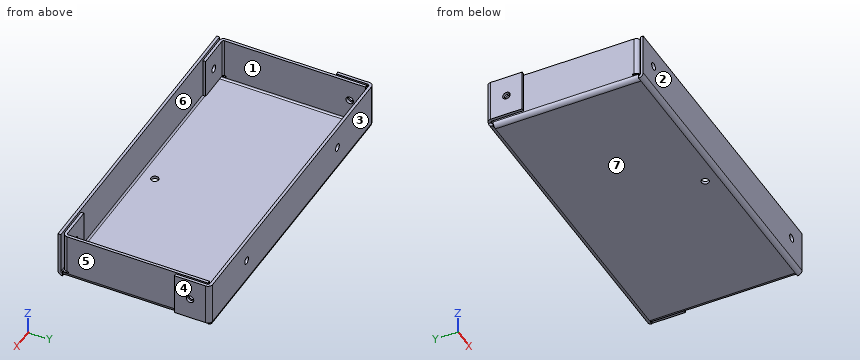
```python
from build123d import *

# Parameters (mm, degrees)
SKETCH1_W                        = 140
SKETCH1_H                        = 70
BASE_FLANGE1_DEPTH               = 1.29
EDGE_FLANGE1_STRIP_W             = 6.684
EDGE_FLANGE1_STRIP_H             = 1.29
EDGE_FLANGE1_STRIP_CUT_DEPTH     = 140
EDGE_FLANGE1_DEPTH               = 140
EDGE_FLANGE2_STRIP_W             = 6.684
EDGE_FLANGE2_STRIP_H             = 1.29
EDGE_FLANGE2_STRIP_CUT_DEPTH     = 140
EDGE_FLANGE2_DEPTH               = 140
EDGE_FLANGE3_STRIP_W             = 6.684
EDGE_FLANGE3_STRIP_H             = 1.29
EDGE_FLANGE3_STRIP_CUT_DEPTH     = 65.896
EDGE_FLANGE3_DEPTH               = 65.896
EDGE_FLANGE4_STRIP_W             = 6.684
EDGE_FLANGE4_STRIP_H             = 1.29
EDGE_FLANGE4_STRIP_CUT_DEPTH     = 65.896
EDGE_FLANGE4_DEPTH               = 65.896
EDGE_FLANGE6_START               = 1.117
EDGE_FLANGE6_DEPTH               = 18.883
EDGE_FLANGE6_2_DEPTH             = 0.645
EDGE_FLANGE6_START_2             = 1.762
EDGE_FLANGE6_3_DEPTH             = 18.238
EDGE_FLANGE8_START               = 1.117
EDGE_FLANGE8_DEPTH               = 18.883
EDGE_FLANGE8_2_DEPTH             = 0.645
EDGE_FLANGE8_START_2             = 1.762
EDGE_FLANGE8_3_DEPTH             = 18.238
M3_CLEARANCE_HOLE1_D             = 3.4
EDGE_FLANGE9_DEPTH               = 19.238
EDGE_FLANGE10_DEPTH              = 19.238
TAP_DRILL_FOR_M4X0_7_TAP1_REACH  = 161.621
TAP_DRILL_FOR_M4X0_7_TAP1_BORE_R = 1.65
M3_CLEARANCE_HOLE3_D             = 3.4
M3_CLEARANCE_HOLE3_DEPTH         = 3.342
M3_CLEARANCE_HOLE4_D             = 3.4


# Read off the part's stored shape, not the designer's step: Edge-Flange6, Edge-Flange8
# Sheet-metal steps are written as plain solids
with BuildPart() as part:
    # Sketch1 → Base-Flange1 (new body)
    with BuildSketch(Plane.XY):
        with Locations((70, 35)):
            Rectangle(SKETCH1_W, SKETCH1_H)
    extrude(amount=-BASE_FLANGE1_DEPTH)

    # Edge-Flange1 strip (across the edge) → Edge-Flange1 strip cut (cut)
    with BuildSketch(Plane(origin=(140, 70, 0), x_dir=(0, -1, 0), z_dir=(-1, 0, 0))):
        with Locations((-1.29, -0.645)):
            Rectangle(EDGE_FLANGE1_STRIP_W, EDGE_FLANGE1_STRIP_H)
    extrude(amount=EDGE_FLANGE1_STRIP_CUT_DEPTH, mode=Mode.SUBTRACT)

    # Edge-Flange1 section (across the edge) → Edge-Flange1 (add)
    with BuildSketch(Plane(origin=(140, 70, 0), x_dir=(0, -1, 0), z_dir=(-1, 0, 0))):
        with BuildLine():
            Line((0, 0.762), (0, 20))
            Line((0, 20), (1.29, 20))
            Line((1.29, 20), (1.29, 0.762))
            ThreePointArc((1.29, 0.762), (1.513184633, 0.223184633), (2.052, 0))
            Line((2.052, 0), (2.052, -1.29))
            ThreePointArc((2.052, -1.29), (0.601016885, -0.688983115), (0, 0.762))
        make_face()
    extrude(amount=EDGE_FLANGE1_DEPTH)

    # Edge-Flange2 strip (across the edge) → Edge-Flange2 strip cut (cut)
    with BuildSketch(Plane.YZ):
        with Locations((-1.29, -0.645)):
            Rectangle(EDGE_FLANGE2_STRIP_W, EDGE_FLANGE2_STRIP_H)
    extrude(amount=EDGE_FLANGE2_STRIP_CUT_DEPTH, mode=Mode.SUBTRACT)

    # Edge-Flange2 section (across the edge) → Edge-Flange2 (add)
    with BuildSketch(Plane.YZ):
        with BuildLine():
            Line((0, 0.762), (0, 20))
            Line((0, 20), (1.29, 20))
            Line((1.29, 20), (1.29, 0.762))
            ThreePointArc((1.29, 0.762), (1.513184633, 0.223184633), (2.052, 0))
            Line((2.052, 0), (2.052, -1.29))
            ThreePointArc((2.052, -1.29), (0.601016885, -0.688983115), (0, 0.762))
        make_face()
    extrude(amount=EDGE_FLANGE2_DEPTH)

    # Edge-Flange3 strip (across the edge) → Edge-Flange3 strip cut (cut)
    with BuildSketch(Plane.XZ.offset(-67.948)):
        with Locations((-1.29, -0.645)):
            Rectangle(EDGE_FLANGE3_STRIP_W, EDGE_FLANGE3_STRIP_H)
    extrude(amount=EDGE_FLANGE3_STRIP_CUT_DEPTH, mode=Mode.SUBTRACT)

    # Edge-Flange3 section (across the edge) → Edge-Flange3 (add)
    with BuildSketch(Plane.XZ.offset(-67.948)):
        with BuildLine():
            Line((0, 0.762), (0, 20))
            Line((0, 20), (1.29, 20))
            Line((1.29, 20), (1.29, 0.762))
            ThreePointArc((1.29, 0.762), (1.513184633, 0.223184633), (2.052, 0))
            Line((2.052, 0), (2.052, -1.29))
            ThreePointArc((2.052, -1.29), (0.601016885, -0.688983115), (0, 0.762))
        make_face()
    extrude(amount=EDGE_FLANGE3_DEPTH)

    # Edge-Flange4 strip (across the edge) → Edge-Flange4 strip cut (cut)
    with BuildSketch(Plane(origin=(140, 2.052, 0), x_dir=(-1, 0, 0), z_dir=(0, 1, 0))):
        with Locations((-1.29, -0.645)):
            Rectangle(EDGE_FLANGE4_STRIP_W, EDGE_FLANGE4_STRIP_H)
    extrude(amount=EDGE_FLANGE4_STRIP_CUT_DEPTH, mode=Mode.SUBTRACT)

    # Edge-Flange4 section (across the edge) → Edge-Flange4 (add)
    with BuildSketch(Plane(origin=(140, 2.052, 0), x_dir=(-1, 0, 0), z_dir=(0, 1, 0))):
        with BuildLine():
            Line((0, 0.762), (0, 20))
            Line((0, 20), (1.29, 20))
            Line((1.29, 20), (1.29, 0.762))
            ThreePointArc((1.29, 0.762), (1.513184633, 0.223184633), (2.052, 0))
            Line((2.052, 0), (2.052, -1.29))
            ThreePointArc((2.052, -1.29), (0.601016885, -0.688983115), (0, 0.762))
        make_face()
    extrude(amount=EDGE_FLANGE4_DEPTH)

    # Edge-Flange6 outline → Edge-Flange6 (cut)
    with BuildSketch(Plane.XY.offset(EDGE_FLANGE6_START)):
        with BuildLine():
            Line((1.29, 2.052), (1.29, 2.198728366))
            ThreePointArc((1.29, 2.198728366), (0.352834322, 2.953547915), (0, 4.104))
            Line((0, 4.104), (0, 2.052))
            Line((0, 2.052), (1.29, 2.052))
        make_face()
    extrude(amount=EDGE_FLANGE6_DEPTH, mode=Mode.SUBTRACT)

    # Edge-Flange6 2 outline → Edge-Flange6 2 (cut)
    with BuildSketch(Plane.XY.offset(EDGE_FLANGE6_START)):
        with BuildLine():
            ThreePointArc((0, 4.104), (0.352834322, 2.953547915), (1.29, 2.198728366))
            Line((1.29, 2.198728366), (1.29, 4.749))
            Line((1.29, 4.749), (0, 4.749))
            Line((0, 4.749), (0, 4.104))
        make_face()
    extrude(amount=EDGE_FLANGE6_2_DEPTH, mode=Mode.SUBTRACT)

    # Edge-Flange6 3 outline → Edge-Flange6 3 (add)
    with BuildSketch(Plane.XY.offset(EDGE_FLANGE6_START_2)):
        with BuildLine():
            Line((2.052, 2.052), (16.29, 2.052))
            Line((16.29, 2.052), (16.29, 3.342))
            Line((16.29, 3.342), (2.052, 3.342))
            ThreePointArc((2.052, 3.342), (1.513184633, 3.565184633), (1.29, 4.104))
            Line((1.29, 4.104), (1.29, 2.198728366))
            ThreePointArc((1.29, 2.198728366), (1.664000898, 2.089015956), (2.052, 2.052))
        make_face()
    extrude(amount=EDGE_FLANGE6_3_DEPTH)

    # Edge-Flange8 outline → Edge-Flange8 (cut)
    with BuildSketch(Plane.XY.offset(EDGE_FLANGE8_START)):
        with BuildLine():
            ThreePointArc((140, 4.104), (139.647165678, 2.953547915), (138.71, 2.198728366))
            Line((138.71, 2.198728366), (138.71, 2.052))
            Line((138.71, 2.052), (140, 2.052))
            Line((140, 2.052), (140, 4.104))
        make_face()
    extrude(amount=EDGE_FLANGE8_DEPTH, mode=Mode.SUBTRACT)

    # Edge-Flange8 2 outline → Edge-Flange8 2 (cut)
    with BuildSketch(Plane.XY.offset(EDGE_FLANGE8_START)):
        with BuildLine():
            Line((138.71, 4.749), (138.71, 2.198728366))
            ThreePointArc((138.71, 2.198728366), (139.647165678, 2.953547915), (140, 4.104))
            Line((140, 4.104), (140, 4.749))
            Line((140, 4.749), (138.71, 4.749))
        make_face()
    extrude(amount=EDGE_FLANGE8_2_DEPTH, mode=Mode.SUBTRACT)

    # Edge-Flange8 3 outline → Edge-Flange8 3 (add)
    with BuildSketch(Plane.XY.offset(EDGE_FLANGE8_START_2)):
        with BuildLine():
            Line((123.71, 2.052), (137.948, 2.052))
            ThreePointArc((137.948, 2.052), (138.335999102, 2.089015956), (138.71, 2.198728366))
            Line((138.71, 2.198728366), (138.71, 4.104))
            ThreePointArc((138.71, 4.104), (138.486815367, 3.565184633), (137.948, 3.342))
            Line((137.948, 3.342), (123.71, 3.342))
            Line((123.71, 3.342), (123.71, 2.052))
        make_face()
    extrude(amount=EDGE_FLANGE8_3_DEPTH)

    # M3 Clearance Hole1 (through all)
    with Locations(Plane(origin=(34.266060613, 19.783275694, -1.29), x_dir=(-1, 0, 0), z_dir=(0, 0, -1))):
        with Locations((-35.733939387, -11.902275694)):
            Hole(M3_CLEARANCE_HOLE1_D / 2)

    # Edge-Flange9 section (across the edge) → Edge-Flange9 (add)
    with BuildSketch(Plane(origin=(140.762, 68.71, 0.762), x_dir=(-1, 0, 0), z_dir=(0, 0, 1))):
        with BuildLine():
            Line((-1.29, 0.762), (-1.29, 15))
            Line((-1.29, 15), (0, 15))
            Line((0, 15), (0, 0.762))
            ThreePointArc((0, 0.762), (0.223184633, 0.223184633), (0.762, 0))
            Line((0.762, 0), (0.762, -1.29))
            ThreePointArc((0.762, -1.29), (-0.688983115, -0.688983115), (-1.29, 0.762))
        make_face()
    extrude(amount=EDGE_FLANGE9_DEPTH)

    # Edge-Flange10 section (across the edge) → Edge-Flange10 (add)
    with BuildSketch(Plane(origin=(-0.762, 68.71, 20), x_dir=(1, 0, 0), z_dir=(0, 0, -1))):
        with BuildLine():
            Line((-1.29, 0.762), (-1.29, 15))
            Line((-1.29, 15), (0, 15))
            Line((0, 15), (0, 0.762))
            ThreePointArc((0, 0.762), (0.223184633, 0.223184633), (0.762, 0))
            Line((0.762, 0), (0.762, -1.29))
            ThreePointArc((0.762, -1.29), (-0.688983115, -0.688983115), (-1.29, 0.762))
        make_face()
    extrude(amount=EDGE_FLANGE10_DEPTH)

    # Tap Drill for M4x0.7 Tap1 bore → Tap Drill for M4x0.7 Tap1 (cut, up to next)
    with BuildSketch(Plane(origin=(0, 70, 0), x_dir=(1, 0, 0), z_dir=(0, 1, 0)), mode=Mode.PRIVATE) as tap_drill_for_m4x0_7_tap1_sk1:
        with Locations((30, -10.381)):
            Circle(TAP_DRILL_FOR_M4X0_7_TAP1_BORE_R)
    tap_drill_for_m4x0_7_tap1_tool1 = extrude(tap_drill_for_m4x0_7_tap1_sk1.sketch, amount=-TAP_DRILL_FOR_M4X0_7_TAP1_REACH, mode=Mode.PRIVATE) & part.part
    # Tap Drill for M4x0.7 Tap1 bore → Tap Drill for M4x0.7 Tap1 (cut, up to next)
    with BuildSketch(Plane(origin=(0, 70, 0), x_dir=(1, 0, 0), z_dir=(0, 1, 0)), mode=Mode.PRIVATE) as tap_drill_for_m4x0_7_tap1_sk2:
        with Locations((110, -10.381)):
            Circle(TAP_DRILL_FOR_M4X0_7_TAP1_BORE_R)
    tap_drill_for_m4x0_7_tap1_tool2 = extrude(tap_drill_for_m4x0_7_tap1_sk2.sketch, amount=-TAP_DRILL_FOR_M4X0_7_TAP1_REACH, mode=Mode.PRIVATE) & part.part
    add(tap_drill_for_m4x0_7_tap1_tool1.solids().sort_by_distance((30, 70, 10.381))[0], mode=Mode.SUBTRACT)
    add(tap_drill_for_m4x0_7_tap1_tool2.solids().sort_by_distance((110, 70, 10.381))[0], mode=Mode.SUBTRACT)

    # M3 Clearance Hole3
    with Locations(Plane(origin=(0, 3.342, 0), x_dir=(1, 0, 0), z_dir=(0, 1, 0))):
        with Locations((9.171, -10.881), (130.829, -10.881)):
            Hole(M3_CLEARANCE_HOLE3_D / 2, depth=M3_CLEARANCE_HOLE3_DEPTH)

    # M3 Clearance Hole4 (through all)
    with Locations(Plane(origin=(142.052, 0, 0), x_dir=(0, 0, -1), z_dir=(1, 0, 0))):
        with Locations((-10.381, 60.829)):
            Hole(M3_CLEARANCE_HOLE4_D / 2)


solid = part.part
```
Geometry: final body of the model. Coordinates: model frame, mm. Face numbers are marked on the shaded views. A direction names the side the tool comes from. Coordinates: 2 decimals unless noted, no trailing zeros. Order: outer loops, then holes, each group sorted by start corner. A loop starts at its lowest first (then second) coordinate and runs counter-clockwise, first axis right, second up. Notation, with made-up numbers: (29.25, 59) - (77.25, 59) arc R33 cw to (77.25, 87) - close; hole circle Ø3 at (88.25, -37.75). An arc over 180 degrees is marked (long way). Return JSON: item names as keys, results as strings. Group by question number.
1. Set-up query: the marked faces 5, 6 and 7. Return all of +Z, -Z, +X, -X, +Y, -Y with unobstructed straight access to the full face (end or side cutting, diameter ignored); none if empty.
2. Cut plane A-A (x = 70). Output: boundary loops of the cut face in (y, z).
3. Pull-direction query (Y, two-part tool) for the marked faces 1, 2, 3 and 4; classes: pulls with the +Y half, pulls with the -Y half, needs draft (parallel to the pull), parting line crosses it, or undercut.
4. Material intervals for line 1 along Y through (x, z) = (6, 8.5); line 2 along X through (y, z) = (48.5, 11); line 3 along Y through (x, z) = (35.5, 17), sorted ascending. Write a range as [from, to].
5. Cut plane C-C (x = 94). Output: boundary loops of the cut face in (y, z), plus the area to 3 significant figures.
6. Cut plane D-D (x = 30). Output: boundary loops of the cut face in (y, z).
7. Cut plane B-B (z = 5.75). Count the separate pieces of the cut face and the enclosed holes in it, plus the area to 3 significant figures.
8. Pin query (flat end, axial travel): pin 1 (1 mm diameter, centred on x = 141.5, y = 63.5, fed in from -Z); pin 2 (3 mm diameter, centred on x = 42, y = 44, fed in from +Z); pin 3 (1.4 mm diameter, centred on x = -1.5, z = 12, fed in from -Y). Return the tip coordinate at first contact, or that it passes through.
Resolved:
{
 "1": {"face 5": "+Z, -Z, -Y", "face 6": "+Z, +X, -X", "face 7": "-Z, +X, -X, +Y, -Y"},
 "2": {"outline": "(0, 0.76) arc R2.05 ccw to (2.05, -1.29) - (6.18, -1.29) - (6.18, 0) - (2.05, 0) arc R0.76 cw to (1.29, 0.76) - (1.29, 20) - (0, 20) - close; (9.58, -1.29) - (67.95, -1.29) arc R2.05 ccw to (70, 0.76) - (70, 20) - (68.71, 20) - (68.71, 0.76) arc R0.76 cw to (67.95, 0) - (9.58, 0) - close"},
 "3": {"face 1": "undercut", "face 2": "pulls with the -Y half", "face 3": "pulls with the +Y half", "face 4": "needs draft"},
 "4": {"line 1": "y = [0, 1.29], [2.05, 3.34], [68.71, 70]", "line 2": "x = [0, 1.29], [138.71, 140]", "line 3": "y = [0, 1.29], [68.71, 70]"},
 "5": {"outline": "(0, 0.76) arc R2.05 ccw to (2.05, -1.29) - (67.95, -1.29) arc R2.05 ccw to (70, 0.76) - (70, 20) - (68.71, 20) - (68.71, 0.76) arc R0.76 cw to (67.95, 0) - (2.05, 0) arc R0.76 cw to (1.29, 0.76) - (1.29, 20) - (0, 20) - close", "area": "140 mm²"},
 "6": {"outline": "(0, 0.76) arc R2.05 ccw to (2.05, -1.29) - (67.95, -1.29) arc R2.05 ccw to (70, 0.76) - (70, 8.73) - (68.71, 8.73) - (68.71, 0.76) arc R0.76 cw to (67.95, 0) - (2.05, 0) arc R0.76 cw to (1.29, 0.76) - (1.29, 20) - (0, 20) - close; (68.71, 12.03) - (70, 12.03) - (70, 20) - (68.71, 20) - close"},
 "7": {"separate pieces": "4", "enclosed holes": "0", "area": "611 mm²"},
 "8": {"pin 1": "stops at z = 0.76", "pin 2": "stops at z = 0", "pin 3": "stops at y = 53.71"}
}
